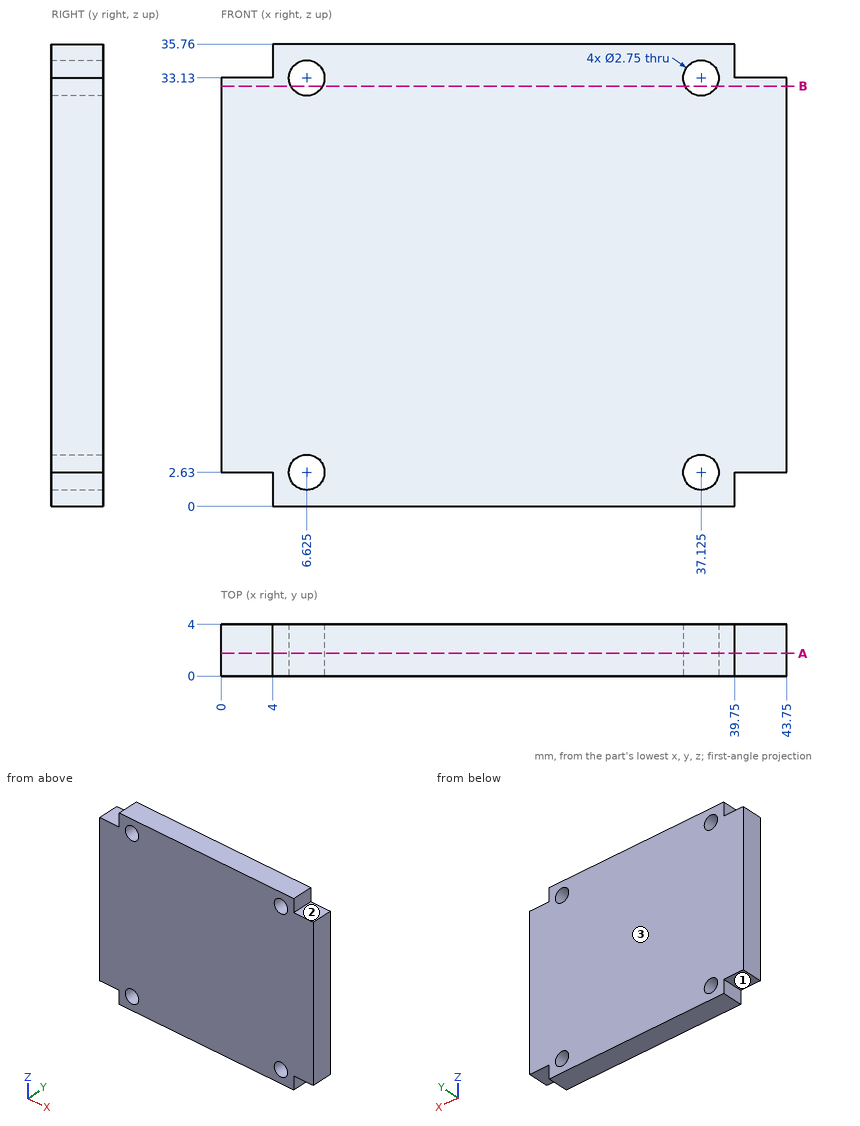
The figure shows three views and two pictorial views of one solid part (mm, origin at its lowest corner). Answer the questions. A direction names the side the tool comes from. Give positions to 0.01 mm unless a question says otherwise; leave off trailing zeros. Order: outer loops, then holes, each group sorted by start corner. A loop starts at its lowest first (then second) coordinate and runs counter-clockwise, first axis right, second up. Notation, with made-up numbers: (28.25, 38) -> (60.25, 38) arc R27 cw to (60.25, 76) -> close; hole circle Ø7 at (7, 44). An arc over 180 degrees is marked (long way). Answer as a JSON object with one key per item and string values. Group by question number.
Item 1: Flat-ended cylindrical pins translate along their axes: pin 1 (0.8 mm diameter, centred on y = 2, z = 34, fed in from -X); pin 2 (2.5 mm diameter, centred on x = 6.625, z = 2.63, fed in from -Y); pin 3 (2 mm diameter, centred on x = 42.5, y = 1, fed in from +Z). Find the tip coordinate at first contact, or state that the pin passes through.
Item 2: Consider L1, parallel to X at y = 1.4, z = 33; L2, parallel to Z at x = 6, y = 2.4; L3, parallel to Z at x = 3.5, y = 1.75. Determine where each line is inside the solid, lowest interval first. Write a range as from..to.
Item 3: The part is cut by section B-B on z = 32.5. Write down the section's boundary in (x, y), and give its area (3 significant figures).
Item 4: A tool of negligible diameter and unlimited length cuts with its end or side. For the marked faces 1, 2 and 3, from which of +Z, -Z, +X, -X, +Y, -Y can it reach the whole face along a straight path? Write none if from no direction.
Item 5: The part is cut by section A-A on y = 1.75. Write down the section's boundary in (x, z) (3 decimals), and give its area (3 significant figures).
Result set:
{
 "1": {"pin 1": "x = 4", "pin 2": "through", "pin 3": "z = 33.13"},
 "2": {"L1": "0..5.26, 7.99..35.76, 38.49..43.75", "L2": "0..1.41, 3.85..31.91, 34.35..35.76", "L3": "2.63..33.13"},
 "3": {"outline": "(0, 0) -> (5.4, 0) -> (5.4, 4) -> (0, 4) -> close; (7.85, 0) -> (35.9, 0) -> (35.9, 4) -> (7.85, 4) -> close; (38.35, 0) -> (43.75, 0) -> (43.75, 4) -> (38.35, 4) -> close", "area": "155 mm²"},
 "4": {"face 1": "-Z, -X, +Y, -Y", "face 2": "+Z, +X, +Y, -Y", "face 3": "+Z, -Z, +X, -X, +Y"},
 "5": {"outline": "(0, 2.63) -> (4, 2.63) -> (4, 0) -> (39.75, 0) -> (39.75, 2.63) -> (43.75, 2.63) -> (43.75, 33.13) -> (39.75, 33.13) -> (39.75, 35.76) -> (4, 35.76) -> (4, 33.13) -> (0, 33.13) -> close; hole circle Ø2.75 at (6.625, 2.63); hole circle Ø2.75 at (6.625, 33.13); hole circle Ø2.75 at (37.125, 2.63); hole circle Ø2.75 at (37.125, 33.13)", "area": "1,500 mm²"}
}
